Design review of the part built by this model. Coordinates are the model's own, in mm. Face numbers are marked on the shaded views. A direction names the side the tool comes from. Coordinates: 2 decimals unless noted, no trailing zeros. Loops run counter-clockwise (first coordinate to the right, second up) from the corner with the lowest first, then second, coordinate; pieces in that order, holes last. Notation, with made-up numbers: M -18.5,75.25 L 2.5,75.25 A13 cw 2.5,84.25 Z; hole C 37.25,-27 d5. An arc over 180 degrees is marked long. Answer as a JSON object with one key per item and string values. Group by question number.
1. Consider section B-B (x = 331). State the section outline as (y, z) points.
2. To check wall thickness, follow probe 1 along Z at (x, y) = (250, 85); probe 2 along X at (y, z) = (90.5, 0); probe 3 along X at (y, z) = (81.5, -102.5). State the ranges of each line that lie inside material, in increasing order.
3. Consider section A-A (y = 83). State the section outline as (x, z) points.
4. Draft analysis for pull direction X (two halves, no side actions). For the marked faces 1, 2, 3 and 4, state which applies: +X half, -X half, draft (parallel to the pull), parting line (faces both ways), or undercut.
5. Insertion check: pin 1 (10 mm diameter, centred on y = 62, z = -52, fed in from -X); pin 2 (12 mm diameter, centred on x = 83, y = 89.5, fed in from +Z); pin 3 (10 mm diameter, centred on y = 53, z = 71.5, fed in from -X). Each pin has a flat end and moves straight along its axis. Give the tip position at first contact, or say it passes through.
6. Consider section D-D (z = -58.5). State the section outline as (x, y) points.
7. Machinability: for the marked faces 5, 6, 7 and 8, which of the approach directions +Z, -Z, +X, -X, +Y, -Y give a long, thin tool a straight path to every point of the face, cutting with its end or side? Answer none if there is none.
8. Consider section C-C (y = 10). State the section outline as (x, z) points, then the cut area to 3 significant figures.
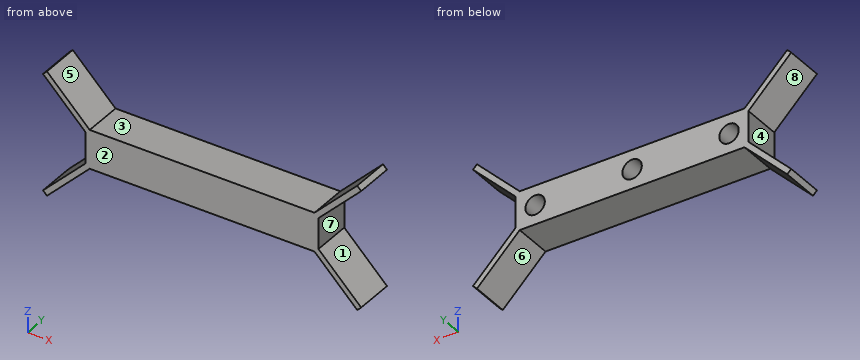
Autodesk Inventor part; units mm, degrees
ref_plane "YZ Plane" through (0, 0, 0) normal (1, 0, 0) x (0, 1, 0)
ref_plane "XZ Plane" through (0, 0, 0) normal (0, 1, 0) x (-1, 0, 0)
ref_plane "XY Plane" through (0, 0, 0) normal (0, 0, 1) x (1, 0, 0)
sketch "Sketch1" plane through (0, 0, 0) normal (0, 1, 0) x (-1, 0, 0)
  line L0 (-300, 50) -> (300, 50)
  line L1 (300, 50) -> (300, -50)
  line L2 (300, -50) -> (-300, -50)
  line L3 (-300, -50) -> (-300, 50)
  line L4 (-300, 50) -> (300, -50) construction
  line L5 (300, 50) -> (-300, -50) construction
  point P0 (0, 0)
  dimension "d0" = 100
  dimension "d1" = 600
extrude "Extrusion1" add sketch "Sketch1" along normal blind 100
sketch "Sketch2" plane through (0, 100, 0) normal (0, 1, 0) x (1, 0, 0)
  line L0 (300, 50) -> (-300, 50)
  line L1 (-300, 50) -> (-400, 150) construction
  line L2 (-410.2193, 150) -> (-300, 39.7807)
  line L3 (-300, 39.7807) -> (-289.7807, 50)
  line L4 (-289.7807, 50) -> (-400, 160.2193)
  line L5 (-400, 160.2193) -> (-410.2193, 150)
  line L6 (-410.2193, 150) -> (-289.7807, 50) construction
  line L7 (-300, 39.7807) -> (-400, 160.2193) construction
  point P0 (0, 0)
  point P1 (-350, 100)
  dimension "d4" = 135
  dimension "d5" = 100
  dimension "d6" = 135
extrude "Extrusion2" add sketch "Sketch2" against normal up to surface (100 mm away)
mirror "Mirror1" about plane through (0, 0, 0) normal (1, 0, 0) of "Extrusion2"
mirror "Mirror2" about plane through (0, 0, 0) normal (0, 0, 1) of "Extrusion2", "Mirror1"
sketch "Sketch4" plane through (0, 100, 0) normal (0, 1, 0) x (1, 0, 0)
  circle A0 centre (0, 0) radius 25
  line L0 (-300, 39.7807) -> (-300, -39.7807) construction
  line L1 (-300, 0) -> (300, 0) construction
  line L2 (300, -39.7807) -> (300, 39.7807) construction
  circle A1 centre (250, 0) radius 25
  line L3 (-50, 0) -> (550, 0) construction
  circle A2 centre (-250, 0) radius 25
  line L4 (-550, 0) -> (50, 0) construction
  circle A3 centre (0, 0) radius 25
  line L5 (-300, 0) -> (300, 0) construction
  dimension "d9" = 50
  dimension "d12" = 250
  dimension "d15" = 250
extrude "Extrusion3" cut sketch "Sketch4" against normal blind 50
properties part number "rotational_platform"
Findings below:
{
 "1": {"outline": "M 0,-91.22 L 100,-91.22 L 100,-70.78 L 0,-70.78 Z; M 0,70.78 L 100,70.78 L 100,91.22 L 0,91.22 Z"},
 "2": {"probe 1": "z = -50 to -25, 25 to 50", "probe 2": "x = -300 to -275, -225 to -25, 25 to 225, 275 to 300", "probe 3": "x = -362.72 to -342.28, 342.28 to 362.72"},
 "3": {"outline": "M -410.22,-150 L -400,-160.22 L -289.78,-50 L 289.78,-50 L 400,-160.22 L 410.22,-150 L 300,-39.78 L 300,39.78 L 410.22,150 L 400,160.22 L 289.78,50 L -289.78,50 L -400,160.22 L -410.22,150 L -300,39.78 L -300,-39.78 Z; hole C -250,0 d50; hole C 0,0 d50; hole C 250,0 d50"},
 "4": {"face 1": "+X half", "face 2": "draft", "face 3": "undercut", "face 4": "-X half"},
 "5": {"pin 1": "stops at x = -317.22", "pin 2": "stops at z = 50", "pin 3": "stops at x = -336.72"},
 "6": {"outline": "M -318.72,0 L -298.28,0 L -298.28,100 L -318.72,100 Z; M 298.28,0 L 318.72,0 L 318.72,100 L 298.28,100 Z"},
 "7": {"face 5": "+Z, +Y, -Y", "face 6": "-Z, +Y, -Y", "face 7": "+X, +Y, -Y", "face 8": "-X, +Y, -Y"},
 "8": {"outline": "M -410.22,-150 L -400,-160.22 L -289.78,-50 L 289.78,-50 L 400,-160.22 L 410.22,-150 L 300,-39.78 L 300,39.78 L 410.22,150 L 400,160.22 L 289.78,50 L -289.78,50 L -400,160.22 L -410.22,150 L -300,39.78 L -300,-39.78 Z", "area": "68,800 mm^2"}
}
